Input: part model. Units: mm. Frame: model coordinates. Face numbers are marked on the shaded views. Coordinates: 2 decimals unless noted, no trailing zeros. Loops run counter-clockwise (first coordinate to the right, second up) from the corner with the lowest first, then second, coordinate; pieces in that order, holes last. Notation, with made-up numbers: M 64.5,-5.75 L 123.5,-5.75 A22 cw 123.5,12.25 Z; hole C -25.5,-16 d8. An arc over 180 degrees is marked long. Use a Markdown table: item, result. Add a question column.
1. Section B-B on y = 11.5. Output: boundary loops of the cut face in (x, z).
2. Section D-D on y = 20.5. Output: boundary loops of the cut face in (x, z).
3. Section A-A on z = -3. Output: boundary loops of the cut face in (x, y), then the cut area to 3 significant figures.
4. Section C-C on x = 9.5. Output: boundary loops of the cut face in (y, z).
5. Line query: L1, parallel to X at y = 8, z = 19.5; L2, parallel to Z at x = 2, y = 20; L3, parallel to Y at x = -39.5, z = -24.5. Output: solid intervals per line, ascending. Write a range as [from, to].
6. Draft query along X for the marked faces 1, 2, 3 and 4. Return one class per face: +X half, -X half, draft (parallel to the pull), parting line (faces both ways), or undercut.
7. Pin query (flat end, axial travel): pin 1 (8 mm diameter, centred on x = 28.448, z = 23.114, fed in from +Y); pin 2 (1.1 mm diameter, centred on x = -74.5, y = 21.5, fed in from -Z); pin 3 (2.5 mm diameter, centred on x = -72, z = 1, fed in from +Y). Return the tip coordinate at first contact, or that it passes through.
```python
from build123d import *

# Parameters (mm, degrees)
SKETCH1_W           = 152.4
SKETCH1_H           = 88.9
BOSS_EXTRUDE1_DEPTH = 38.1
SKETCH2_W           = 147.32
SKETCH2_H           = 83.82
CUT_EXTRUDE1_DEPTH  = 33.02
SKETCH5_W           = 9.398
SKETCH5_H           = 3.429
CUT_EXTRUDE3_DEPTH  = 2.54
FILLET1_R           = 2.54
SKETCH6_R           = 2.54
CUT_EXTRUDE4_DEPTH  = 95.194282735
SKETCH7_W           = 10.16
SKETCH7_H           = 4.572
SKETCH7_W_2         = 9.398
SKETCH7_H_2         = 3.556
BOSS_EXTRUDE2_DEPTH = 3.048


with BuildPart() as part:
    # Sketch1 → Boss-Extrude1 (new body)
    with BuildSketch(Plane(origin=(0, 0, 0), x_dir=(1, 0, 0), z_dir=(0, 1, 0))):
        Rectangle(SKETCH1_W, SKETCH1_H)
    extrude(amount=BOSS_EXTRUDE1_DEPTH)

    # Sketch2 → Cut-Extrude1 (cut)
    with BuildSketch(Plane(origin=(0, 38.1, 0), x_dir=(1, 0, 0), z_dir=(0, 1, 0))):
        Rectangle(SKETCH2_W, SKETCH2_H)
    extrude(amount=-CUT_EXTRUDE1_DEPTH, mode=Mode.SUBTRACT)

    # Sketch5 → Cut-Extrude3 (cut)
    with BuildSketch(Plane.ZY.offset(76.2)):
        with Locations((0, 20.574)):
            Rectangle(SKETCH5_W, SKETCH5_H)
    extrude(amount=-CUT_EXTRUDE3_DEPTH, mode=Mode.SUBTRACT)

    # Fillet1
    fillet1_edges = [part.edges().sort_by_distance(p)[0] for p in [
        (76.2, 19.05, 44.45),
        (-76.2, 19.05, 44.45),
        (-76.2, 19.05, -44.45),
        (76.2, 19.05, -44.45),
    ]]
    fillet(fillet1_edges, radius=FILLET1_R)

    # Sketch6 → Cut-Extrude4 (cut, through all)
    with BuildSketch(Plane(origin=(0, 5.08, 0), x_dir=(1, 0, 0), z_dir=(0, 1, 0))):
        with Locations(Location((28.448, 23.114, 0), (0, 0, 270))):
            Circle(SKETCH6_R)
        with Locations(Location((28.448, -23.114, 0), (0, 0, 90))):
            Circle(SKETCH6_R)
    extrude(amount=-CUT_EXTRUDE4_DEPTH, mode=Mode.SUBTRACT)

    # Sketch7 → Boss-Extrude2 (add)
    with BuildSketch(Plane(origin=(-73.66, 0, 0), x_dir=(0, 0, -1), z_dir=(1, 0, 0))):
        with Locations((0, 20.5105)):
            Rectangle(SKETCH7_W, SKETCH7_H)
        with Locations((0, 20.5105)):
            Rectangle(SKETCH7_W_2, SKETCH7_H_2, mode=Mode.SUBTRACT)
    extrude(amount=BOSS_EXTRUDE2_DEPTH)


solid = part.part
```
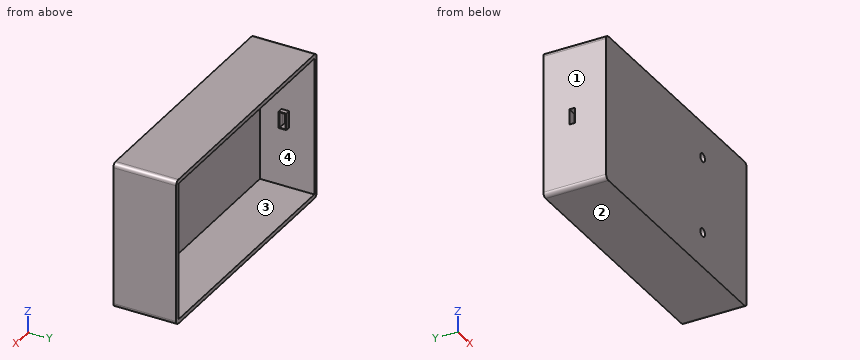
Answers below:
| question | item | result |
|---|---|---|
| 1 | outline | M -76.2,-41.91 A2.54 ccw -73.66,-44.45 L 73.66,-44.45 A2.54 ccw 76.2,-41.91 L 76.2,41.91 A2.54 ccw 73.66,44.45 L -73.66,44.45 A2.54 ccw -76.2,41.91 Z; hole M -73.66,-41.91 L 73.66,-41.91 L 73.66,41.91 L -73.66,41.91 Z |
| 2 | outline | M -76.2,-41.91 A2.54 ccw -73.66,-44.45 L 73.66,-44.45 A2.54 ccw 76.2,-41.91 L 76.2,41.91 A2.54 ccw 73.66,44.45 L -73.66,44.45 A2.54 ccw -76.2,41.91 L -76.2,4.7 L -70.61,4.7 L -70.61,5.08 L -73.66,5.08 L -73.66,41.91 L 73.66,41.91 L 73.66,-41.91 L -73.66,-41.91 L -73.66,-5.08 L -70.61,-5.08 L -70.61,-4.7 L -76.2,-4.7 Z |
| 3 | outline | M -76.2,0 L 76.2,0 L 76.2,38.1 L 73.66,38.1 L 73.66,5.08 L -73.66,5.08 L -73.66,18.22 L -70.61,18.22 L -70.61,18.73 L -73.66,18.73 L -73.66,18.86 L -76.2,18.86 Z; M -76.2,22.29 L -70.61,22.29 L -70.61,22.8 L -73.66,22.8 L -73.66,38.1 L -76.2,38.1 Z |
| 3 | area | 936 mm² |
| 4 | outline | M 0,-44.45 L 38.1,-44.45 L 38.1,-41.91 L 5.08,-41.91 L 5.08,41.91 L 38.1,41.91 L 38.1,44.45 L 0,44.45 Z |
| 5 | L1 | x = [-76.2, -73.66], [73.66, 76.2] |
| 5 | L2 | z = [-44.45, -41.91], [41.91, 44.45] |
| 5 | L3 | y = [0, 5.08] |
| 6 | face 1 | -X half |
| 6 | face 2 | draft |
| 6 | face 3 | undercut |
| 6 | face 4 | undercut |
| 7 | pin 1 | stops at y = 5.08 |
| 7 | pin 2 | stops at z = -44.43 |
| 7 | pin 3 | stops at y = 22.8 |
